from build123d import *

# Parameters (mm, degrees)
F0_W     = 152.4
F0_H     = 88.9
F1_DEPTH = 101.6
F3_DEPTH = 152.4
F4_W     = 50.8
F4_H     = 9.9303191528
F5_DEPTH = 12.7
F6_W     = 38.1
F6_H     = 6.35
F7_DEPTH = 25.4
F8_T     = -7.62


with BuildPart() as f1:
    # F0 (on Top) → F1 (new body)
    with BuildSketch(Plane.XY):
        with Locations((-1.1791149259, -0.9629391849)):
            Rectangle(F0_W, F0_H)
    extrude(amount=F1_DEPTH)

    # F2 (on face) → F3 (join)
    with BuildSketch(Plane.YZ.offset(75.0208850741)):
        Polygon((-14.8739154544, 114.1574053684), (-45.4129391849, 101.6), (43.4870608151, 101.6), (12.9480370846, 114.1574053684), align=None)
    extrude(amount=-F3_DEPTH)

    # F4 (on face) → F5 (join)
    with BuildSketch(Plane.XY.offset(114.1574053684)):
        with Locations((-1.1791149259, -2.587900497)):
            Rectangle(F4_W, F4_H)
    extrude(amount=F5_DEPTH)

    # F6 (on face) → F7 (cut)
    with BuildSketch(Plane.XZ.offset(7.5530600734)):
        with Locations((-1.1791149259, 117.3324053684)):
            Rectangle(F6_W, F6_H)
    extrude(amount=-F7_DEPTH, mode=Mode.SUBTRACT)

    # F8
    f8_openings = [f1.faces().sort_by_distance(p)[0] for p in [
        (-1.179115, -0.962939, 0),
    ]]
    offset(amount=F8_T, openings=f8_openings, kind=Kind.INTERSECTION)


solid = f1.part
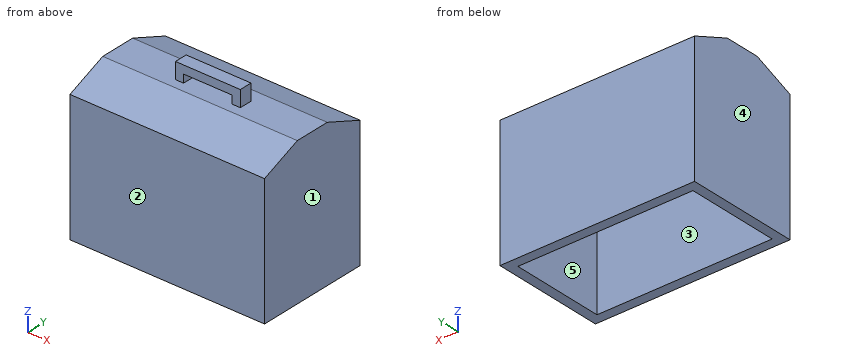
Geometry: final body of the model. Coordinates: model frame, mm. Face numbers are marked on the shaded views. A direction names the side the tool comes from. Coordinates: 2 decimals unless noted, no trailing zeros. Loops run counter-clockwise (first coordinate to the right, second up) from the corner with the lowest first, then second, coordinate; pieces in that order, holes last. Notation, with made-up numbers: M 84,82 L 117,82 A26 ccw 117,108 Z; hole C 52,69.25 d6. An arc over 180 degrees is marked long. One line per item, written item: value. Start each with the question number.
1) Reachability of the marked faces 4 and 5 from +Z, -Z, +X, -X, +Y, -Y: full face, straight path, thin tool, end or side. Return the list, or none.
2) Material intervals for L1, parallel to X at y = 11, z = 26; L2, parallel to Y at x = -69, z = 64; L3, parallel to Z at x = -4, y = -6, sorted ascending. Write a range as from..to.
3) Pin query (flat end, axial travel): P1, Ø1.9, axis at y = -0.5, z = 118.5, coming from the -X side; P2, Ø5, axis at x = -2.5, y = -2, coming from the -Z side; P3, Ø14, axis at x = -1, z = 119.5, coming from the +Y side. Return the tip coordinate at first contact, or that it passes through.
4) Cut plane D-D (y = 6.5). Return loops of the section in (x, z).
5) Cut plane B-B (z = 31.5). Return loops of the section in (x, y).
6) Cut plane C-C (x = 20.5). Return loops of the section in (y, z).
7) Cut plane A-A (x = -8.5). Return loops of the section in (y, z).
8) Draft query along Y for the marked faces 1, 2 and 3. Return one class per face: released by +Y, released by -Y, zero draft, split by the parting line, or undercut.
Evaluation:
1. face 4: +Z, -Z, -X, +Y, -Y
1. face 5: -Z
2. L1: -77.38..-69.76, 67.4..75.02
2. L2: -45.41..-37.79, 35.87..43.49
2. L3: 106.54..114.16, 120.51..126.86
3. P1: x = -26.58
3. P2: z = 106.54
3. P3: y = 16.98
4. outline: M -77.38,0 L -69.76,0 L -69.76,106.54 L 67.4,106.54 L 67.4,0 L 75.02,0 L 75.02,114.16 L -77.38,114.16 Z
5. outline: M -77.38,-45.41 L 75.02,-45.41 L 75.02,43.49 L -77.38,43.49 Z; hole M -69.76,-37.79 L 67.4,-37.79 L 67.4,35.87 L -69.76,35.87 Z
6. outline: M -45.41,0 L -37.79,0 L -37.79,96.49 L -13.37,106.54 L 11.44,106.54 L 35.87,96.49 L 35.87,0 L 43.49,0 L 43.49,101.6 L 12.95,114.16 L 2.38,114.16 L 2.38,126.86 L -7.55,126.86 L -7.55,114.16 L -14.87,114.16 L -45.41,101.6 Z
7. outline: M -45.41,0 L -37.79,0 L -37.79,96.49 L -13.37,106.54 L 11.44,106.54 L 35.87,96.49 L 35.87,0 L 43.49,0 L 43.49,101.6 L 12.95,114.16 L -14.87,114.16 L -45.41,101.6 Z; M -7.55,120.51 L 2.38,120.51 L 2.38,126.86 L -7.55,126.86 Z
8. face 1: zero draft
8. face 2: released by -Y
8. face 3: undercut
